```python
from build123d import *

# Parameters (mm, degrees)
BOSS_EXTRUDE2_DEPTH     = 12.7
SKETCH4_R               = 10.419425035
BOSS_EXTRUDE3_DEPTH     = 12.7
CUT_EXTRUDE1_DEPTH      = 144.616730223
CUT_EXTRUDE1_DEPTH_BACK = 144.616730223
SKETCH3_R               = 6.35


with BuildPart() as part:
    # Sketch2 → Boss-Extrude2 (new body)
    with BuildSketch(Plane.XY):
        with BuildLine():
            Line((0, 15.24), (127, 15.24))
            ThreePointArc((127, 15.24), (142.24, 0), (127, -15.24))
            Line((127, -15.24), (0, -15.24))
            ThreePointArc((0, -15.24), (-15.24, 0), (0, 15.24))
        make_face()
    extrude(amount=BOSS_EXTRUDE2_DEPTH)

    # Sketch4 → Boss-Extrude3 (add)
    with BuildSketch(Plane.XY.offset(12.7)):
        Circle(SKETCH4_R)
    extrude(amount=BOSS_EXTRUDE3_DEPTH)

    # Sketch3 → Cut-Extrude1 (cut, two sides: drawn at the far end of the back side and taken through both)
    with BuildSketch(Plane.XY.offset(12.7).offset(-CUT_EXTRUDE1_DEPTH_BACK)):
        Circle(SKETCH3_R)
        with Locations((127, 0)):
            Circle(SKETCH3_R)
    extrude(amount=CUT_EXTRUDE1_DEPTH + CUT_EXTRUDE1_DEPTH_BACK, mode=Mode.SUBTRACT)


solid = part.part
```
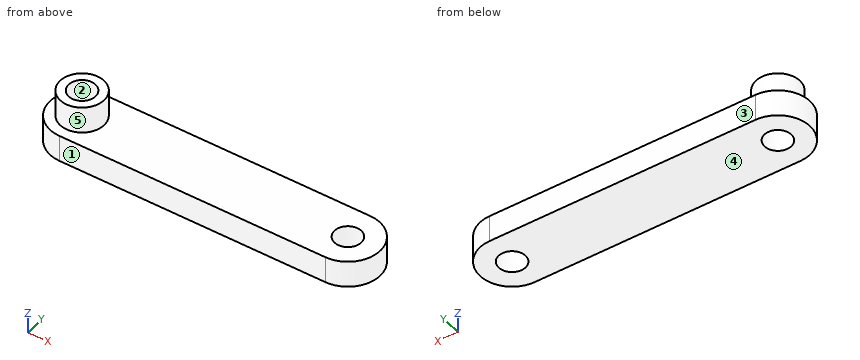
Geometry: final body of the model. Coordinates: model frame, mm. Face numbers are marked on the shaded views. A direction names the side the tool comes from. Coordinates: 2 decimals unless noted, no trailing zeros. Order: outer loops, then holes, each group sorted by start corner. A loop starts at its lowest first (then second) coordinate and runs counter-clockwise, first axis right, second up. Notation, with made-up numbers: (-0.75, 34.25) - (32.25, 34.25) arc R26 ccw to (32.25, 66.25) - close; hole circle Ø3 at (2, -12). An arc over 180 degrees is marked (long way). Write each question's results on one line, items separated by ' | '.
(1) Section query C-C, the plane z = 21.5. Return the cut outline in (x, y), plus the area to 3 significant figures.
Values found:
outline: circle Ø20.84 at (0, 0); hole circle Ø12.7 at (0, 0) | area: 214 mm²
(2) Line query: line 1 (X direction, y = 0.5, z = 10); line 2 (Z direction, x = 96, y = -3.5); line 3 (X direction, y = 4, z = 5.5). Output: solid intervals per line, ascending. Write a range as [from, to].
Values found:
line 1: x = [-15.23, -6.33], [6.33, 120.67], [133.33, 142.23] | line 2: z = [0, 12.7] | line 3: x = [-14.71, -4.93], [4.93, 122.07], [131.93, 141.71]
(3) Section query A-A, the plane z = 8. Return the cut outline in (x, y).
Values found:
outline: (0, -15.24) - (127, -15.24) arc R15.24 ccw to (127, 15.24) - (0, 15.24) arc R15.24 ccw to start; hole circle Ø12.7 at (0, 0); hole circle Ø12.7 at (127, 0)
(4) Section query B-B, the plane y = 0. Return the cut outline in (x, z), plus the area to 3 significant figures.
Values found:
outline: (-15.24, 0) - (-6.35, 0) - (-6.35, 25.4) - (-10.42, 25.4) - (-10.42, 12.7) - (-15.24, 12.7) - close; (6.35, 0) - (120.65, 0) - (120.65, 12.7) - (10.42, 12.7) - (10.42, 25.4) - (6.35, 25.4) - close; (133.35, 0) - (142.24, 0) - (142.24, 12.7) - (133.35, 12.7) - close | area: 1,780 mm²
(5) Section query D-D, the plane x = 114. Return the cut outline in (y, z).
Values found:
outline: (-15.24, 0) - (15.24, 0) - (15.24, 12.7) - (-15.24, 12.7) - close
(6) Mould query, pull axis Y, two halves, no side actions, for the marked faces 1, 2 and 3. Classes: +Y half, -Y half, draft (parallel to the pull), parting line (faces both ways), or undercut.
Values found:
face 1: -Y half | face 2: undercut | face 3: +Y half
(7) Set-up query: the marked faces 4 and 5. Return all of +Z, -Z, +X, -X, +Y, -Y with unobstructed straight access to the full face (end or side cutting, diameter ignored); none if empty.
Values found:
face 4: -Z, +X, -X, +Y, -Y | face 5: +Z
(8) First-contact query: pin 1 Ø10 at (x, y) = (103, -6) entering from +Z; pin 2 Ø3 at (y, z) = (8, 17) entering from -X; pin 3 Ø2 at (y, z) = (-6.5, 7) entering from +X. Flat tips, straight axial feed; report the tip coordinate or a pass-through.
Values found:
pin 1: stops at z = 12.7 | pin 2: stops at x = -8.14 | pin 3: stops at x = 141.21
